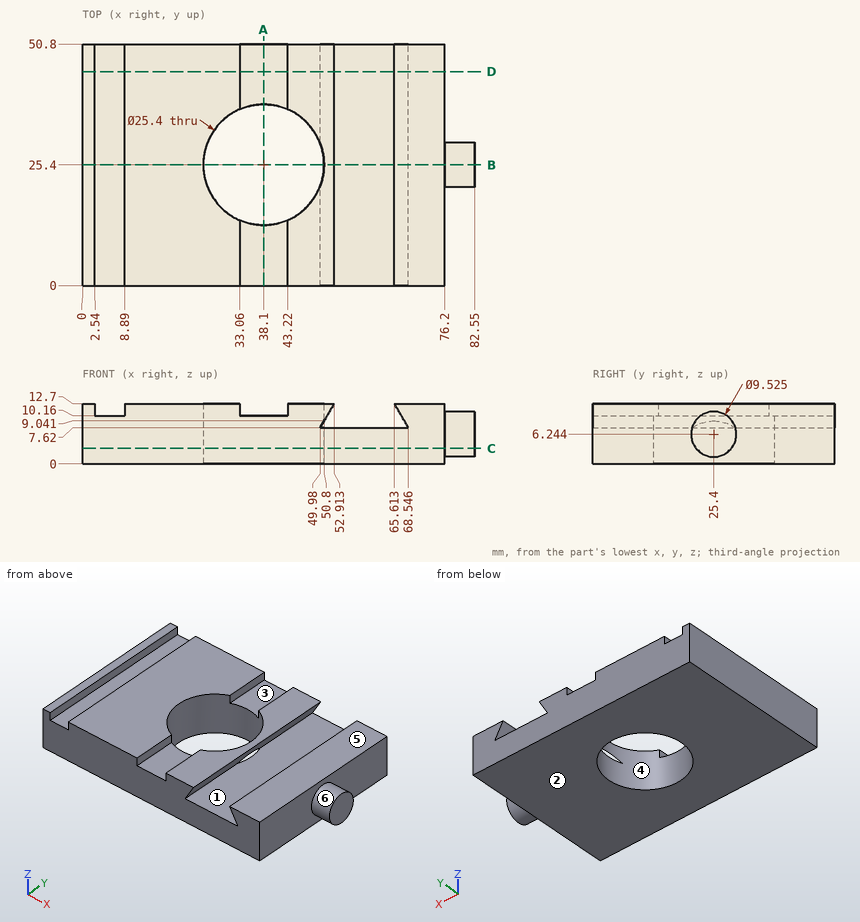
Study the drawing (mm; zero at the part's minimum x, y, z) and answer. A direction names the side the tool comes from. Coordinates: 2 decimals unless noted, no trailing zeros. Loops run counter-clockwise (first coordinate to the right, second up) from the corner with the lowest first, then second, coordinate; pieces in that order, holes last. Notation, with made-up numbers: (-28, 68.5) -> (24, 68.5) arc R24 ccw to (24, 91.5) -> close; hole circle Ø10 at (-1.75, 65). An arc over 180 degrees is marked (long way). Answer as CSV lines item,"result".
1) The part is cut by section A-A (x = 38.1). Give the vertices of the cut face in (y, z), and give its area (3 significant figures).
A:
outline,"(0, 0) -> (12.7, 0) -> (12.7, 10.16) -> (0, 10.16) -> close; (38.1, 0) -> (50.8, 0) -> (50.8, 10.16) -> (38.1, 10.16) -> close"
area,"258 mm²"
2) Straight lines are drawn through the part: probe 1 along Y at (x, z) = (38.1, 4); probe 2 along X at (y, z) = (30, 8.5); probe 3 along X at (y, z) = (16.5, 9.5) (1 decimal). For each, find the intervals that lie inside material, in ascending order.
A:
probe 1,"y = 0 to 12.7, 38.1 to 50.8"
probe 2,"x = 0 to 26.26, 49.94 to 50.49, 68.04 to 76.2"
probe 3,"x = 0 to 29, 47.2 to 51.1, 67.5 to 76.2"
3) The part is cut by section B-B (y = 25.4). State how many separate pieces and enclosed holes the cut face has, and give its area (3 significant figures).
A:
separate pieces,"3"
enclosed holes,"0"
area,"611 mm²"
4) The part is cut by section D-D (y = 45). Give the vertices of the cut face in (x, z) (1 decimal).
A:
outline,"(0, 0) -> (76.2, 0) -> (76.2, 12.7) -> (65.6, 12.7) -> (68.5, 7.6) -> (50, 7.6) -> (52.9, 12.7) -> (43.2, 12.7) -> (43.2, 10.2) -> (33.1, 10.2) -> (33.1, 12.7) -> (8.9, 12.7) -> (8.9, 10.2) -> (2.5, 10.2) -> (2.5, 12.7) -> (0, 12.7) -> close"
5) The part is cut by section C-C (z = 3.25). Give the vertices of the cut face in (x, y), and give its area (3 significant figures).
A:
outline,"(0, 0) -> (76.2, 0) -> (76.2, 21.7) -> (82.55, 21.7) -> (82.55, 29.1) -> (76.2, 29.1) -> (76.2, 50.8) -> (0, 50.8) -> close; hole circle Ø25.4 at (38.1, 25.4)"
area,"3,410 mm²"
6) For a pull along Y with two mould halves and no side action, classify the marked faces 4, 5 and 6 as released by +Y, released by -Y, zero draft, split by the parting line, or undercut.
A:
face 4,"undercut"
face 5,"zero draft"
face 6,"split by the parting line"
7) For the marked faces 1, 2 and 3, determine the directions among +Z, -Z, +X, -X, +Y, -Y from which every point of the face is accessible in a straight line to the end or side of a thin tool.
A:
face 1,"+Y, -Y"
face 2,"-Z, +X, -X, +Y, -Y"
face 3,"+Z, +Y, -Y"
8) Flat-ended cylindrical pins translate along their axes: pin 1 (3 mm diameter, centred on y = 30.5, z = 11, fed in from +X); pin 2 (3 mm diameter, centred on x = 37.5, y = 8, fed in from +Z). Find the tip coordinate at first contact, or state that the pin passes through.
A:
pin 1,"stops at x = 76.2"
pin 2,"stops at z = 10.16"
